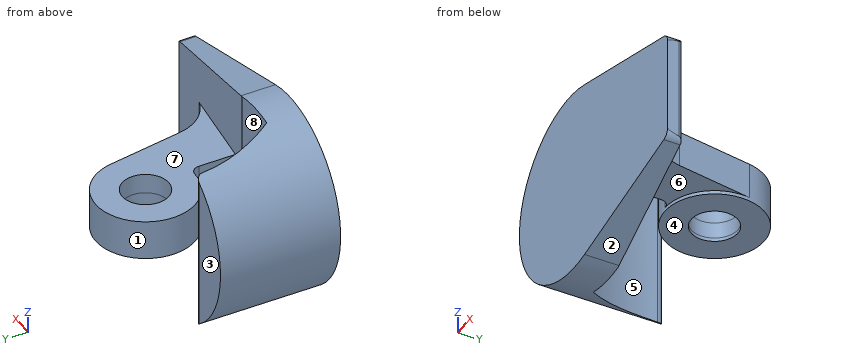
from build123d import *

# Parameters (mm, degrees)
SKETCH1_R                = 10.5
BOSS_EXTRUDE1_DEPTH      = 13.5
CUT_EXTRUDE1_DEPTH       = 11.5
CUT_EXTRUDE1_DEPTH_BACK  = 11.5
SKETCH5_R                = 5.5
SKETCH5_R_2              = 2.575
BOSS_EXTRUDE2_DEPTH      = 2.2
BOSS_EXTRUDE2_DEPTH_BACK = 1.8
SKETCH5_4_R              = 5.5
SKETCH5_4_R_2            = 2.575
BOSS_EXTRUDE3_DEPTH      = 2.2
FILLET1_R                = 1


with BuildPart() as part:
    # Sketch1 → Boss-Extrude1 (new body)
    with BuildSketch(Plane(origin=(0, 0, 0), x_dir=(1, 0, 0), z_dir=(0, 1, 0))):
        with BuildLine():
            Line((18.443804907, 6.19010049), (2.559951525, 10.18315512))
            ThreePointArc((2.559951525, 10.18315512), (8.280383174, 6.45641189), (10.5, 0))
            ThreePointArc((10.5, 0), (8.280383174, -6.45641189), (2.559951525, -10.18315512))
            Line((2.559951525, -10.18315512), (18.443804907, -6.19010049))
            ThreePointArc((18.443804907, -6.19010049), (18.988607921, -5.835172564), (19.2, -5.220276193))
            Line((19.2, -5.220276193), (19.2, 5.220276193))
            ThreePointArc((19.2, 5.220276193), (18.988607921, 5.835172564), (18.443804907, 6.19010049))
        make_face()
        Circle(SKETCH1_R)
    extrude(amount=BOSS_EXTRUDE1_DEPTH)

    # Sketch2 → Cut-Extrude1 (cut, two sides)
    with BuildSketch(Plane.XY) as cut_extrude1_sk:
        with BuildLine():
            Line((-85.748448257, 13.5), (-10.5, 13.5))
            Line((-10.5, 13.5), (-6.28259424, 13.5))
            ThreePointArc((-6.28259424, 13.5), (-5.729347477, 13.277856401), (-5.483351282, 12.73479505))
            ThreePointArc((-5.483351282, 12.73479505), (-4.659552595, 8.127259704), (-2.65, 3.9))
            Line((-2.65, 3.9), (2.253530088, 3.9))
            ThreePointArc((2.253530088, 3.9), (2.349801107, 3.896907442), (2.445675162, 3.887642521))
            Line((2.445675162, 3.887642521), (18.648491256, 1.794874091))
            ThreePointArc((18.648491256, 1.794874091), (18.945201048, 1.645191976), (19.082540247, 1.342571122))
            Line((19.082540247, 1.342571122), (19.2, 0))
            Line((19.2, 0), (25.758334398, -74.962105194))
            Line((25.758334398, -74.962105194), (119.29298444, 42.938637392))
            Line((119.29298444, 42.938637392), (7.786201784, 131.400742585))
            Line((7.786201784, 131.400742585), (-85.748448257, 13.5))
        make_face()
    extrude(amount=CUT_EXTRUDE1_DEPTH, mode=Mode.SUBTRACT)
    extrude(cut_extrude1_sk.sketch, amount=-CUT_EXTRUDE1_DEPTH_BACK, mode=Mode.SUBTRACT)

    # Sketch5 → Boss-Extrude2 (add, two sides)
    with BuildSketch(Plane.XY) as boss_extrude2_sk:
        with BuildLine():
            Line((9.93428712, 6.560044551), (8.528350834, 15.184876952))
            ThreePointArc((8.528350834, 15.184876952), (8.582058445, 14.743886479), (8.6, 14.3))
            ThreePointArc((8.6, 14.3), (7.295235393, 10.743316151), (4, 8.874136013))
            Line((4, 8.874136013), (4, 3.9))
            Line((4, 3.9), (4, 2.282191618))
            Line((4, 2.282191618), (14.2, 2.282191618))
            ThreePointArc((14.2, 2.282191618), (11.37916934, 3.735096256), (9.93428712, 6.560044551))
        make_face()
        with Locations((3.1, 14.3)):
            Circle(SKETCH5_R)
        with Locations((3.1, 14.3)):
            Circle(SKETCH5_R_2, mode=Mode.SUBTRACT)
    extrude(amount=BOSS_EXTRUDE2_DEPTH)
    extrude(boss_extrude2_sk.sketch, amount=-BOSS_EXTRUDE2_DEPTH_BACK)

    # Sketch5<4> → Boss-Extrude3 (add)
    with BuildSketch(Plane.XY):
        with Locations((3.1, 14.3)):
            Circle(SKETCH5_4_R)
        with Locations((3.1, 14.3)):
            Circle(SKETCH5_4_R_2, mode=Mode.SUBTRACT)
    extrude(amount=-BOSS_EXTRUDE3_DEPTH)

    # Fillet1
    fillet1_edges = [part.edges().sort_by_distance(p)[0] for p in [
        (4, 8.874136013, 0.2),
    ]]
    fillet(fillet1_edges, radius=FILLET1_R)


solid = part.part
Part model, mm, in its own coordinate system. Face numbers are marked on the shaded views. A direction names the side the tool comes from. Round coordinates to 2 decimals unless told otherwise and drop trailing zeros. Order: outer loops, then holes, each group sorted by start corner. A loop starts at its lowest first (then second) coordinate and runs counter-clockwise, first axis right, second up. Notation, with made-up numbers: (43.25, -33) -> (97.25, -33) arc R10 ccw to (97.25, -15) -> close; hole circle Ø2 at (48.25, 48.5). An arc over 180 degrees is marked (long way). Put each result on its own line as item: value.
Q1. Wall check: line 1 (Y direction, x = 3.1, z = -1.4) (3 decimals); line 2 (Z direction, x = 1.5, y = 10.5); line 3 (X direction, y = 7, z = 0.5). Give the ranges that are in metal, low to high. Write a range as [from, to].
From the geometry:
line 1: y = [0, 3.803], [8.796, 11.725], [16.875, 19.8]
line 2: z = [-2.2, 2.2]
line 3: x = [-10.49, -4.26], [4, 9.86]
Q2. Band-saw the part on A-A (y = 9.25). Give the cut face in (x, z), and give its area (3 significant figures).
From the geometry:
outline: (-4.98, -9.24) -> (-4.98, 9.24) arc R10.5 ccw to start; (0.92, -2.2) -> (5.28, -2.2) -> (5.28, -1.8) -> (9.5, -1.8) -> (9.5, 2.2) -> (0.92, 2.2) -> close
area: 109 mm2
Q3. Pull direction Y, two halves, no side cores. Call the marked faces 1, 2 and 3: pulls with the +Y half, pulls with the -Y half, needs draft (parallel to the pull), parting line crosses it, or undercut.
From the geometry:
face 1: undercut
face 2: needs draft
face 3: pulls with the +Y half
Q4. Pin check, flat tips, straight feed: pin 1 Ø5 at (y, z) = (10, 5) entering from -X; pin 2 Ø2 at (x, y) = (15.5, 3) entering from -Z; pin 3 Ø4 at (x, z) = (0.5, 1.5) entering from +Y. Stop position of each tip, or through.
From the geometry:
pin 1: stops at x = -10.2
pin 2: stops at z = -7.11
pin 3: stops at y = 19.77
Q5. Band-saw the part on D-D (x = 6.25). Give the cut face in (y, z).
From the geometry:
outline: (0, -9.26) -> (3.4, -9.26) -> (3.4, -1.8) -> (9.79, -1.8) -> (9.79, -2.2) -> (18.81, -2.2) -> (18.81, 2.2) -> (3.4, 2.2) -> (3.4, 9.26) -> (0, 9.26) -> close
Q6. Tool access for the marked faces 4, 5, 6, 7 and 8: list every direction of +Z, -Z, +X, -X, +Y, -Y with a clear straight run to the whole face (end or side of a thin tool).
From the geometry:
face 4: -Z, +X, +Y
face 5: +Z, -Z, +Y
face 6: -Z, +X
face 7: +Z, +X, +Y
face 8: +Z, -Z
Q7. Band-saw the part on B-B (x = 0). Give the cut face in (y, z).
From the geometry:
outline: (0, -10.5) -> (3.9, -10.5) -> (3.9, 10.5) -> (0, 10.5) -> close; (9.76, -2.2) -> (18.84, -2.2) -> (18.84, 2.2) -> (9.76, 2.2) -> close
